Part model, mm, in its own coordinate system. Round coordinates to 2 decimals unless told otherwise and drop trailing zeros. Loops run counter-clockwise (first coordinate to the right, second up) from the corner with the lowest first, then second, coordinate; pieces in that order, holes last. Notation, with made-up numbers: (-37, -10) -> (-22, -10) arc R24 cw to (-22, 25) -> close; hole circle Ø2 at (36, -0.5). An arc over 180 degrees is marked (long way). Use a Markdown table: item, result. Add a question column.
Item 1: Probe line 1 (Z direction, x = 5.5, y = 38.1); line 2 (Y direction, x = 5, z = 54); line 3 (Z direction, x = 3, y = 65.5). List the from-to ranges inside material, lowest first. Write a range as [from, to].
Item 2: Cut at B-B, the plane z = 0. List the corners of the cut face in (x, y), plus the area to 3 significant figures.
Item 3: Cut at C-C, the plane z = -19.05. List the corners of the cut face in (x, y), plus the area to 3 significant figures.
Item 4: Cut at A-A, the plane y = -12.7. List the corners of the cut face in (x, z), plus the area to 3 significant figures.
Item 5: Two-plate mould, pull along Z, no slides. Class faces 1 (the face through (5, -1, 76)), 2 (the face through (0, -18, 1)), 3 (the face through (4.93, -65.828, 21.588)), 4 (the face through (4.93, 60.596, -20.901)): pulls with the +Z half, pulls with the -Z half, needs draft (parallel to the pull), parting line crosses it, or undercut.
Item 6: Cut at D-D, the plane x = 8.25. State how many separate pieces and enclosed holes the cut face has, plus the area to 3 significant figures.
Item 7: Flat gauge pin, fed straight in: pin 1 (4 mm diameter, centred on y = -63.5, z = 19.05, fed in from -X). Where does the tip first touch, or does it go through?
Autodesk Inventor part; units mm, degrees
ref_plane "YZ Plane" through (0, 0, 0) normal (1, 0, 0) x (0, 1, 0)
ref_plane "XZ Plane" through (0, 0, 0) normal (0, 1, 0) x (-1, 0, 0)
ref_plane "XY Plane" through (0, 0, 0) normal (0, 0, 1) x (1, 0, 0)
sketch "Sketch5" plane through (0, 0, 0) normal (1, 0, 0) x (0, 1, 0)
  line L0 (76, -76) -> (-76, -76)
  line L1 (-76, -76) -> (-76, 76)
  line L2 (-76, 76) -> (76, 76)
  line L3 (76, 76) -> (76, -76)
  line L4 (76, -76) -> (-76, 76) construction
  line L5 (-76, -76) -> (76, 76) construction
  point P0 (0, 0)
  dimension "d31" = 152
  dimension "d32" = 152
extrude "Extrusion2" add sketch "Sketch5" along normal blind 10
sketch "Sketch6" plane through (10, 0, 0) normal (1, 0, 0) x (0, 0, -1)
  line L0 (76, -76) -> (76, 76)
  line L1 (76, 76) -> (-76, 76)
  point P0 (0, 0)
  point P1 (50.6, 50.6)
  dimension "d42" = 25.4
  dimension "d43" = 25.4
hole "Hole4" at (10, 50.6, -50.6) direction (-1, 0, 0) diameter 12.7 end through all
sketch "Sketch7" plane through (10, 0, 0) normal (1, 0, 0) x (0, 0, -1)
  circle A0 centre (50.6, 50.6) radius 6.35
  line L0 (76, 76) -> (-76, 76)
  point P0 (0, 0)
  point P1 (-51, 50.6)
  dimension "d51" = 101.6
  dimension "d52" = 25.4
hole "Hole5" at (10, 50.6, 51) direction (-1, 0, 0) diameter 12.7 end through all
sketch "Sketch8" plane through (10, 0, 0) normal (1, 0, 0) x (0, 0, -1)
  line L0 (76, -76) -> (76, 76)
  circle A0 centre (50.6, 50.6) radius 6.35
  point P0 (0, 0)
  point P1 (50.6, -51)
  dimension "d60" = 25.4
  dimension "d61" = 101.6
hole "Hole6" at (10, -51, -50.6) direction (-1, 0, 0) diameter 12.7 end through all
sketch "Sketch9" plane through (10, 0, 0) normal (1, 0, 0) x (0, 0, -1)
  circle A0 centre (-51, 50.6) radius 6.35
  circle A1 centre (50.6, -51) radius 6.35
  point P0 (0, 0)
  point P1 (-51, -51)
  dimension "d69" = 101.6
  dimension "d70" = 101.6
hole "Hole7" at (10, -51, 51) direction (-1, 0, 0) diameter 12.7 end through all
sketch "Sketch10" plane through (10, 0, 0) normal (1, 0, 0) x (0, 0, -1)
  line L0 (76, 76) -> (-76, 76)
  line L1 (76, -76) -> (76, 76)
  point P0 (0, 0)
  point P1 (19.05, 63.5)
  dimension "d93" = 12.5
  dimension "d103" = 56.95
hole "Hole8" at (10, 63.5, -19.05) direction (-1, 0, 0) diameter 6.888 end through all
sketch "Sketch11" plane through (10, 0, 0) normal (1, 0, 0) x (0, 0, -1)
  circle A0 centre (19.05, 63.5) radius 3.444
  point P0 (0, 0)
  point P1 (-19.05, 63.5)
  dimension "d85" = 38.1
  dimension "d86" = 0
hole "Hole9" at (10, 63.5, 19.05) direction (-1, 0, 0) diameter 6.888 end through all
pattern_linear "Rectangular Pattern1" count 6 spacing 25.4 along (0, -1, 0) of "Hole8"
pattern_linear "Rectangular Pattern2" count 6 spacing 25.4 along (0, -1, 0) of "Hole9"
sketch "Sketch12" plane through (10, 0, 0) normal (1, 0, 0) x (0, 0, -1)
  line L0 (76, -76) -> (76, 76)
  line L1 (-76, -76) -> (76, -76)
  point P0 (0, 0)
  point P1 (0, 0)
  dimension "d101" = 76
  dimension "d102" = 76
hole "Hole10" at (10, 0, 0) direction (-1, 0, 0) diameter 5 end through all
properties part number "base_plate"
A:
| question | item | result |
|---|---|---|
| 1 | line 1 | z = [-76, -22.49], [-15.61, 15.61], [22.49, 76] |
| 1 | line 2 | y = [-76, -56.6], [-45.4, 45], [56.2, 76] |
| 1 | line 3 | z = [-76, -21.85], [-16.25, 16.25], [21.85, 76] |
| 2 | outline | (0, -76) -> (10, -76) -> (10, -2.5) -> (0, -2.5) -> close; (0, 2.5) -> (10, 2.5) -> (10, 76) -> (0, 76) -> close |
| 2 | area | 1,470 mm^2 |
| 3 | outline | (0, -76) -> (10, -76) -> (10, -66.94) -> (0, -66.94) -> close; (0, -60.06) -> (10, -60.06) -> (10, -41.54) -> (0, -41.54) -> close; (0, -34.66) -> (10, -34.66) -> (10, -16.14) -> (0, -16.14) -> close; (0, -9.26) -> (10, -9.26) -> (10, 9.26) -> (0, 9.26) -> close; (0, 16.14) -> (10, 16.14) -> (10, 34.66) -> (0, 34.66) -> close; (0, 41.54) -> (10, 41.54) -> (10, 60.06) -> (0, 60.06) -> close; (0, 66.94) -> (10, 66.94) -> (10, 76) -> (0, 76) -> close |
| 3 | area | 1,110 mm^2 |
| 4 | outline | (0, -76) -> (10, -76) -> (10, -22.49) -> (0, -22.49) -> close; (0, -15.61) -> (10, -15.61) -> (10, 15.61) -> (0, 15.61) -> close; (0, 22.49) -> (10, 22.49) -> (10, 76) -> (0, 76) -> close |
| 4 | area | 1,380 mm^2 |
| 5 | face 1 | pulls with the +Z half |
| 5 | face 2 | needs draft |
| 5 | face 3 | undercut |
| 5 | face 4 | undercut |
| 6 | separate pieces | 1 |
| 6 | enclosed holes | 17 |
| 6 | area | 22,100 mm^2 |
| 7 | pin 1 | passes through |
